from build123d import *

# Parameters (mm, degrees)
SKETCH1_R           = 9.6
BASE_EXTRUDE_DEPTH  = 23.7
CUT_EXTRUDE1_DEPTH  = 21.7
BOSS_EXTRUDE1_DEPTH = 16
SKETCH4_R           = 1.3
CUT_EXTRUDE2_DEPTH  = 40.7
FILLET4_R           = 0.4


with BuildPart() as part:
    # Sketch1 → Base-Extrude (new body)
    with BuildSketch(Plane.XY):
        Circle(SKETCH1_R)
    extrude(amount=BASE_EXTRUDE_DEPTH)

    # Sketch2 → Cut-Extrude1 (cut)
    with BuildSketch(Plane(origin=(0, 0, 0), x_dir=(-1, 0, 0), z_dir=(0, 0, -1))):
        with BuildLine():
            Line((1.151331339, 6.016608995), (1.151331339, 4.741608995))
            ThreePointArc((1.151331339, 4.741608995), (3.409837287, 3.474244057), (4.677202225, 1.215738109))
            Line((4.677202225, 1.215738109), (5.952202225, 1.215738109))
            ThreePointArc((5.952202225, 1.215738109), (6.747697354, 0.886233238), (7.077202225, 0.090738109))
            ThreePointArc((7.077202225, 0.090738109), (6.747697354, -0.70475702), (5.952202225, -1.034261891))
            Line((5.952202225, -1.034261891), (4.677202225, -1.034261891))
            ThreePointArc((4.677202225, -1.034261891), (3.409837287, -3.292767839), (1.151331339, -4.560132777))
            Line((1.151331339, -4.560132777), (1.151331339, -5.835132777))
            ThreePointArc((1.151331339, -5.835132777), (0.026331339, -6.960132777), (-1.098668661, -5.835132777))
            Line((-1.098668661, -5.835132777), (-1.098668661, -4.560132777))
            ThreePointArc((-1.098668661, -4.560132777), (-3.357174609, -3.292767839), (-4.624539548, -1.034261891))
            Line((-4.624539548, -1.034261891), (-5.899539548, -1.034261891))
            ThreePointArc((-5.899539548, -1.034261891), (-6.695034676, -0.70475702), (-7.024539548, 0.090738109))
            ThreePointArc((-7.024539548, 0.090738109), (-6.695034676, 0.886233238), (-5.899539548, 1.215738109))
            Line((-5.899539548, 1.215738109), (-4.624539548, 1.215738109))
            ThreePointArc((-4.624539548, 1.215738109), (-3.357174609, 3.474244057), (-1.098668661, 4.741608995))
            Line((-1.098668661, 4.741608995), (-1.098668661, 6.016608995))
            ThreePointArc((-1.098668661, 6.016608995), (-0.76916379, 6.812104124), (0.026331339, 7.141608995))
            ThreePointArc((0.026331339, 7.141608995), (0.821826467, 6.812104124), (1.151331339, 6.016608995))
        make_face()
    extrude(amount=-CUT_EXTRUDE1_DEPTH, mode=Mode.SUBTRACT)

    # Sketch3 → Boss-Extrude1 (add)
    with BuildSketch(Plane.XY.offset(23.7)):
        with BuildLine():
            Line((-1.151331339, 6.016608995), (-1.151331339, 4.741608995))
            ThreePointArc((-1.151331339, 4.741608995), (-3.409837287, 3.474244057), (-4.677202225, 1.215738109))
            Line((-4.677202225, 1.215738109), (-5.952202225, 1.215738109))
            ThreePointArc((-5.952202225, 1.215738109), (-6.747697354, 0.886233238), (-7.077202225, 0.090738109))
            ThreePointArc((-7.077202225, 0.090738109), (-6.747697354, -0.70475702), (-5.952202225, -1.034261891))
            Line((-5.952202225, -1.034261891), (-4.677202225, -1.034261891))
            ThreePointArc((-4.677202225, -1.034261891), (-3.409837287, -3.292767839), (-1.151331339, -4.560132777))
            Line((-1.151331339, -4.560132777), (-1.151331339, -5.835132777))
            ThreePointArc((-1.151331339, -5.835132777), (-0.026331339, -6.960132777), (1.098668661, -5.835132777))
            Line((1.098668661, -5.835132777), (1.098668661, -4.560132777))
            ThreePointArc((1.098668661, -4.560132777), (3.357174609, -3.292767839), (4.624539548, -1.034261891))
            Line((4.624539548, -1.034261891), (5.899539548, -1.034261891))
            ThreePointArc((5.899539548, -1.034261891), (6.695034676, -0.70475702), (7.024539548, 0.090738109))
            ThreePointArc((7.024539548, 0.090738109), (6.695034676, 0.886233238), (5.899539548, 1.215738109))
            Line((5.899539548, 1.215738109), (4.624539548, 1.215738109))
            ThreePointArc((4.624539548, 1.215738109), (3.357174609, 3.474244057), (1.098668661, 4.741608995))
            Line((1.098668661, 4.741608995), (1.098668661, 6.016608995))
            ThreePointArc((1.098668661, 6.016608995), (0.76916379, 6.812104124), (-0.026331339, 7.141608995))
            ThreePointArc((-0.026331339, 7.141608995), (-0.821826467, 6.812104124), (-1.151331339, 6.016608995))
        make_face()
    extrude(amount=BOSS_EXTRUDE1_DEPTH)

    # Sketch4 → Cut-Extrude2 (cut, through all)
    with BuildSketch(Plane.XY.offset(39.7)):
        with Locations((-0.026331339, 0.090738109)):
            Circle(SKETCH4_R)
    extrude(amount=-CUT_EXTRUDE2_DEPTH, mode=Mode.SUBTRACT)

    # Sketch5 → Cut-Revolve1 (revolve, cut)
    with BuildSketch(Plane(origin=(0, 0, 0), x_dir=(0, 0, -1), z_dir=(1, 0, 0))):
        Polygon((0, 9.6), (-23.7, 9.4), (-23.7, 9.6), align=None)
    revolve(axis=Axis((0, 0, 0), (0, 0, 1)), mode=Mode.SUBTRACT)

    # Fillet4
    fillet4_edges = [part.edges().sort_by_distance(p)[0] for p in [
        (0, -9.4, 23.7),
        (-5.314702225, 1.215738109, 39.7),
        (-1.151331339, -5.197632777, 39.7),
        (1.098668661, -5.197632777, 39.7),
        (5.262039548, -1.034261891, 39.7),
        (1.098668661, 5.379108995, 39.7),
        (-0.026331339, 7.141608995, 39.7),
        (-1.151331339, 5.379108995, 39.7),
        (-3.409837287, 3.474244057, 39.7),
        (-7.077202225, 0.090738109, 39.7),
        (-5.314702225, -1.034261891, 39.7),
        (-3.409837287, -3.292767839, 39.7),
        (-0.026331339, -6.960132777, 39.7),
        (3.357174609, -3.292767839, 39.7),
        (7.024539548, 0.090738109, 39.7),
        (5.262039548, 1.215738109, 39.7),
        (3.357174609, 3.474244057, 39.7),
    ]]
    fillet(fillet4_edges, radius=FILLET4_R)


solid = part.part
For this review, take the finished solid that the model builds, in its own axes (mm). A direction names the side the tool comes from. Round coordinates to 2 decimals unless told otherwise and drop trailing zeros. Write each loop counter-clockwise with the first axis right and the second up, starting at its lowest first coordinate (ties: lowest second). Pieces come first, ordered by that corner, then holes. Notation, with made-up numbers: (56, 9.25) - (71, 9.25) arc R25 cw to (71, 40.25) - close; hole circle Ø7 at (72, 49.25). An arc over 180 degrees is marked (long way). Write item = value, one per line. Start each with the question number.
1. Consider section B-B on z = 11. State the section outline as (x, y) points (3 decimals).
2. Draft analysis for pull direction Y (two halves, no side actions). For faces 6 (the face through (-1.151, 5, 31)), 7 (the face through (3.33, -3.32, 31.39)), 8 (the face through (1.099, -5, 11)), 9 (the face through (-5, -1.034, 11)), state which applies: released by +Y, released by -Y, zero draft, split by the parting line, or undercut.
3. Wall thickness on L1, parallel to Z at x = 3.25, y = -4; L2, parallel to Y at x = 6.75, z = 13.5; L3, parallel to X at y = 1, z = 10: over which ranges is each line inside the solid? List them lowest first.
4. For pin 1 Ø1.5 at (y, z) = (2.5, 33.5) entering from -X; pin 2 Ø6 at (x, y) = (-1, -7) entering from +Z; pin 3 Ø0.6 at (x, z) = (5, 9) entering from -Y; pin 4 Ø0.6 at (x, z) = (-5, 9) entering from +Y, all flat-tipped, find the tip position at first contact; note any pin that passes through.
5. Consider section A-A on z = 35. State the section outline as (x, y) points (3 decimals), plus the area to 3 significant figures.
6. For faces 1 (the face through (4, -4, 0)), 2 (the face through (5, 1.216, 11)), 3 (the face through (1.099, -5, 31)), 4 (the face through (-5, 1.216, 31)), 5 (the face through (-5, -1.034, 31)), list the 3-axis set-ups (+Z, -Z, +X, -X, +Y, -Y) from which the entire face can be reached by the end or side of a thin tool; tool diameter is ignored.
Evaluation:
q1.outline = circle Ø19.014 at (0, 0); hole (-5.952, -1.034) - (-4.677, -1.034) arc R4.785 ccw to (-1.151, -4.56) - (-1.151, -5.835) arc R1.125 ccw to (1.099, -5.835) - (1.099, -4.56) arc R4.785 ccw to (4.625, -1.034) - (5.9, -1.034) arc R1.125 ccw to (5.9, 1.216) - (4.625, 1.216) arc R4.785 ccw to (1.099, 4.742) - (1.099, 6.017) arc R1.125 ccw to (-1.151, 6.017) - (-1.151, 4.742) arc R4.785 ccw to (-4.677, 1.216) - (-5.952, 1.216) arc R1.125 ccw to start
q2.face_6 = zero draft
q2.face_7 = released by -Y
q2.face_8 = undercut
q2.face_9 = undercut
q3.L1 = 0 to 23.7
q3.L2 = -6.67 to -0.65, 0.83 to 6.67
q3.L3 = -9.46 to -6.61, 6.56 to 9.46
q4.pin_1 = -4.51
q4.pin_2 = 39.7
q4.pin_3 = -8.28
q4.pin_4 = 8.28
q5.outline = (-5.952, -1.034) - (-4.677, -1.034) arc R4.785 ccw to (-1.151, -4.56) - (-1.151, -5.835) arc R1.125 ccw to (1.099, -5.835) - (1.099, -4.56) arc R4.785 ccw to (4.625, -1.034) - (5.9, -1.034) arc R1.125 ccw to (5.9, 1.216) - (4.625, 1.216) arc R4.785 ccw to (1.099, 4.742) - (1.099, 6.017) arc R1.125 ccw to (-1.151, 6.017) - (-1.151, 4.742) arc R4.785 ccw to (-4.677, 1.216) - (-5.952, 1.216) arc R1.125 ccw to start; hole circle Ø2.6 at (-0.026, 0.091)
q5.area = 85.2 mm2
q6.face_1 = -Z, +X, -X, +Y, -Y
q6.face_2 = -Z
q6.face_3 = +Z, +X, -Y
q6.face_4 = +Z, -X, +Y
q6.face_5 = +Z, -X, -Y
